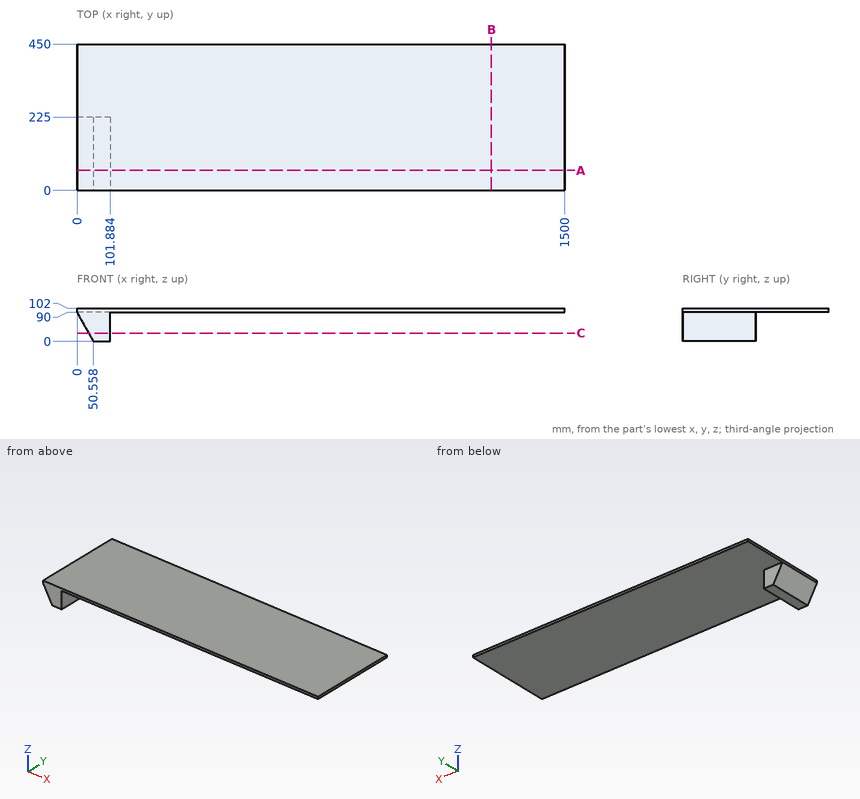
Print and shaded views of the part. All mm, measured from the part's lowest x, y and z. Round coordinates to 2 decimals unless told otherwise and drop trailing zeros. Write each loop counter-clockwise with the first axis right and the second up, starting at its lowest first coordinate (ties: lowest second). Pieces come first, ordered by that corner, then holes. Notation, with made-up numbers: (-35.75, -13.5) -> (10.25, -13.5) arc R27 ccw to (10.25, 9.5) -> close; hole circle Ø1 at (70, -13). An arc over 180 degrees is marked (long way). Return JSON: item names as keys, results as strings. Group by question number.
Q1. Saw through at C-C on z = 26. Write the cut outline in (x, y), plus the area to 3 significant figures.
Q2. Saw through at A-A on y = 61.5. Write the cut outline in (x, z), plus the area to 3 significant figures.
Q3. Probe L1, parallel to Z at x = 384.5, y = 66; L2, parallel to X at y = 104.5, z = 11 (1 decimal); L3, parallel to X at y = 104.5, z = 16.5 (1 decimal). List the from-to ranges inside material, lowest first. Write a range as [from, to].
Q4. Pin check, flat tips, straight feed: pin 1 (3 mm diameter, centred on y = 126.5, z = 81, fed in from -X); pin 2 (8 mm diameter, centred on x = 227, z = 86.5, fed in from -Y); pin 3 (8 mm diameter, centred on x = 1147.5, y = 380.5, fed in from -Z); pin 4 (6 mm diameter, centred on y = 160, z = 49, fed in from -X). Stop position of each tip, or through.
Q5. Saw through at B-B on x = 1274.5. Write the cut outline in (y, z), plus the area to 3 significant figures.
Answer:
{
 "1": {"outline": "(35.95, 0) -> (101.88, 0) -> (101.88, 225) -> (35.95, 225) -> close", "area": "14,800 mm2"},
 "2": {"outline": "(0, 90) -> (50.56, 0) -> (101.88, 0) -> (101.88, 90) -> (1500, 90) -> (1500, 102) -> (0, 102) -> close", "area": "24,900 mm2"},
 "3": {"L1": "[90, 102]", "L2": "[44.4, 101.9]", "L3": "[41.3, 101.9]"},
 "4": {"pin 1": "x = 4.21", "pin 2": "y = 0", "pin 3": "z = 90", "pin 4": "x = 21.35"},
 "5": {"outline": "(0, 90) -> (450, 90) -> (450, 102) -> (0, 102) -> close", "area": "5,400 mm2"}
}
